from build123d import *

# Parameters (mm, degrees)
F0_W     = 120
F0_H     = 120
F1_DEPTH = 1300
F2_W     = 40
F2_H     = 175
F3_DEPTH = 120
F4_R     = 5.25
F5_DEPTH = 120.001
F6_R     = 5.25
F7_DEPTH = 120.001


with BuildPart() as f1:
    # F0 (on Top) → F1 (new body, symmetric)
    with BuildSketch(Plane.XY):
        Rectangle(F0_W, F0_H)
    extrude(amount=F1_DEPTH, both=True)

    # F2 (on face) → F3 (cut, through all)
    with BuildSketch(Plane.YZ.offset(60)):
        with Locations((-40, 1212.5)):
            Rectangle(F2_W, F2_H)
    extrude(amount=-F3_DEPTH, mode=Mode.SUBTRACT)

    # F4 (on face) → F5 (cut, through all)
    with BuildSketch(Plane(origin=(0, 60, 0), x_dir=(-1, 0, 0), z_dir=(0, 1, 0))):
        with Locations((0, 1212.5)):
            Circle(F4_R)
        with Locations((0, -900)):
            Circle(F4_R)
        with Locations((0, 600)):
            Circle(F4_R)
    extrude(amount=-F5_DEPTH, mode=Mode.SUBTRACT)

    # F6 (on face) → F7 (cut, through all)
    with BuildSketch(Plane.YZ.offset(60)):
        with Locations((0, -950)):
            Circle(F6_R)
        with Locations((0, 700)):
            Circle(F6_R)
    extrude(amount=-F7_DEPTH, mode=Mode.SUBTRACT)


solid = f1.part
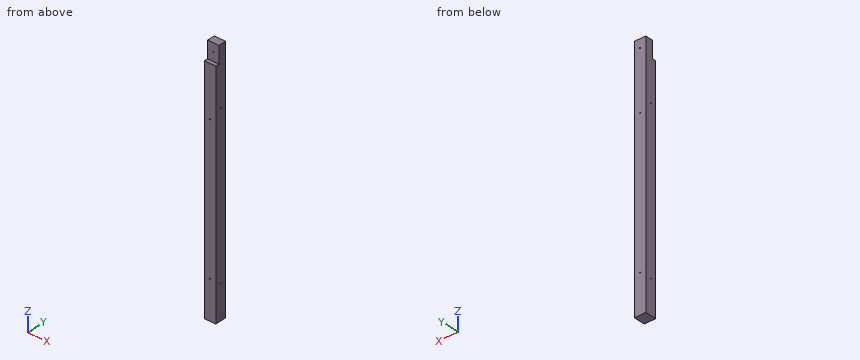
Read the model definition and answer for the solid it produces. Units are mm, in the model's axes. Round coordinates to 2 decimals unless told otherwise and drop trailing zeros. Loops run counter-clockwise (first coordinate to the right, second up) from the corner with the lowest first, then second, coordinate; pieces in that order, holes last.
Q1. Each of these flat-tipped pins is pushed along its axis until it touches: pin 1 (12 mm diameter, centred on x = -28, y = -37.5, fed in from +Z); pin 2 (9.5 mm diameter, centred on x = 0, z = 1212.5, fed in from +Y). Where does it stop, or does it pass through?
Q2. Consider probe 1 along Z at (x, y) = (0, 30.5); probe 2 along Z at (x, y) = (1.5, -51.5); probe 3 along X at (y, z) = (32.5, 600). Determine where each line is inside the solid, lowest interval first.
Q3. Section A-A on x = -38.5 is taken. Write down the section's boundary in (y, z).
Output:
1. pin 1: stops at z = 1125
1. pin 2: passes through
2. probe 1: z = -1300 to -905.25, -894.75 to 594.75, 605.25 to 1207.25, 1217.75 to 1300
2. probe 2: z = -1300 to -905.03, -894.97 to 594.97, 605.03 to 1125
2. probe 3: x = -60 to -5.25, 5.25 to 60
3. outline: (-60, -1300) - (60, -1300) - (60, 1300) - (-20, 1300) - (-20, 1125) - (-60, 1125) - close; hole circle Ø10.5 at (0, -950); hole circle Ø10.5 at (0, 700)
